from build123d import *

# Parameters (mm, degrees)
SKETCH1_R                = 5
BOSS_EXTRUDE1_DEPTH      = 9
BOSS_EXTRUDE1_DEPTH_BACK = 13
SKETCH2_R                = 3
CUT_EXTRUDE1_DEPTH       = 5
SKETCH3_R                = 4
CUT_EXTRUDE2_DEPTH       = 5
SKETCH5_R                = 5
SKETCH5_R_2              = 4.7
CUT_EXTRUDE3_DEPTH       = 0.3
LPATTERN1_COUNT          = 10
LPATTERN1_PITCH          = 1


with BuildPart() as part:
    # Sketch1 → Boss-Extrude1 (new body, two sides)
    with BuildSketch(Plane.XY) as boss_extrude1_sk:
        Circle(SKETCH1_R)
    extrude(amount=BOSS_EXTRUDE1_DEPTH)
    extrude(boss_extrude1_sk.sketch, amount=-BOSS_EXTRUDE1_DEPTH_BACK)

    # Sketch2 → Cut-Extrude1 (cut)
    with BuildSketch(Plane.XY.offset(9)):
        Circle(SKETCH2_R)
    extrude(amount=-CUT_EXTRUDE1_DEPTH, mode=Mode.SUBTRACT)

    # Sketch3 → Cut-Extrude2 (cut)
    with BuildSketch(Plane(origin=(0, 0, -13), x_dir=(-1, 0, 0), z_dir=(0, 0, -1))):
        Circle(SKETCH3_R)
    extrude(amount=-CUT_EXTRUDE2_DEPTH, mode=Mode.SUBTRACT)

    # Sketch5 → Cut-Extrude3 (cut)
    with BuildSketch(Plane.XY):
        Circle(SKETCH5_R)
        Circle(SKETCH5_R_2, mode=Mode.SUBTRACT)
    cut_extrude3 = extrude(amount=-CUT_EXTRUDE3_DEPTH, mode=Mode.SUBTRACT)

    # LPattern1: Cut-Extrude3 ×10
    with Locations(*[(0, 0, -i * LPATTERN1_PITCH) for i in range(1, LPATTERN1_COUNT)]):
        add(cut_extrude3, mode=Mode.SUBTRACT)


solid = part.part
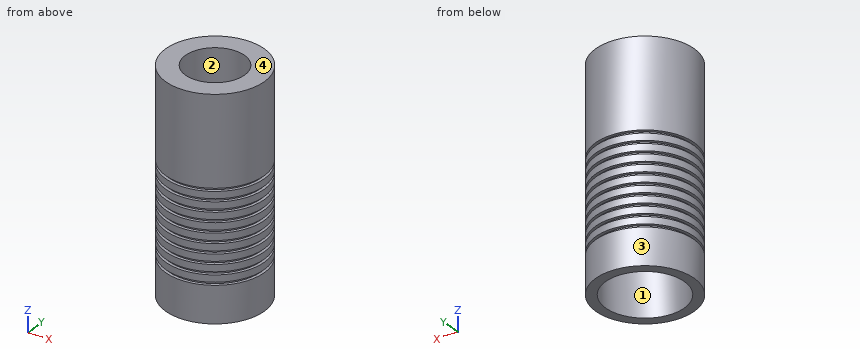
Check sheet for the modelled part. Datum: model origin and axes. Units: mm. Face numbers are marked on the shaded views. Coordinates: 2 decimals unless noted, no trailing zeros. Loops run counter-clockwise (first coordinate to the right, second up) from the corner with the lowest first, then second, coordinate; pieces in that order, holes last. Notation, with made-up numbers: (4.5, 75) -> (44.5, 75) arc R7 ccw to (44.5, 87) -> close; hole circle Ø7 at (70.25, 73.5). An arc over 180 degrees is marked (long way). Answer in a Markdown table with one row per item.
1. Material ranges on line 1 along Y through (x, z) = (0, 7.3); line 2 along Y through (x, z) = (0, -9.5); line 3 along Z through (x, y) = (-3, -0.75), recorded low to high. Write a range as [from, to].
Check values:
| item | result |
|---|---|
| line 1 | y = [-5, -3], [3, 5] |
| line 2 | y = [-5, -4], [4, 5] |
| line 3 | z = [-8, 9] |
2. Release check for a two-part mould opening along X. For the marked faces 1, 2, 3 and 4 record: released by +X, released by -X, zero draft, split by the parting line, or undercut.
Check values:
| item | result |
|---|---|
| face 1 | undercut |
| face 2 | undercut |
| face 3 | split by the parting line |
| face 4 | zero draft |
3. Go/stop test with flat-tipped pins: pin 1 (2 mm diameter, centred on x = -0.5, y = 0.5, fed in from -Z); pin 2 (4 mm diameter, centred on y = -3, z = 5, fed in from +X); pin 3 (2 mm diameter, centred on y = 3.5, z = 4, fed in from +X). Record where each tip stops, or that it passes through.
Check values:
| item | result |
|---|---|
| pin 1 | stops at z = -8 |
| pin 2 | stops at x = 4.9 |
| pin 3 | stops at x = 4.33 |
4. Sectioned sample at A-A, the plane z = 2.5. Record the boundary of the cut face in (x, y).
Check values:
| item | result |
|---|---|
| outline | circle Ø10 at (0, 0) |
